Autodesk Inventor part; units mm, degrees
ref_plane "YZ Plane" through (0, 0, 0) normal (1, 0, 0) x (0, 1, 0)
ref_plane "XZ Plane" through (0, 0, 0) normal (0, 1, 0) x (-1, 0, 0)
ref_plane "XY Plane" through (0, 0, 0) normal (0, 0, 1) x (1, 0, 0)
sketch "Sketch1" plane through (0, 0, 0) normal (0, 1, 0) x (-1, 0, 0)
  point P0 (0, 0)
sketch "Sketch2" plane through (0, 0, 0) normal (0, 0, 1) x (1, 0, 0)
  line L0 (0, 0) -> (0, 25)
  line L1 (0, 25) -> (-5, 25)
  line L2 (-5, 25) -> (-5, 2.5)
  line L3 (-5, 2.5) -> (-85, 2.5)
  line L4 (-85, 2.5) -> (-85, 25)
  line L5 (-85, 25) -> (-90, 25)
  line L6 (-90, 25) -> (-90, 0)
  line L7 (-90, 0) -> (0, 0)
  line L8 (-85, 2.5) -> (-5, 2.5)
  line L9 (-5, 2.5) -> (-5, -2.5)
  line L10 (-5, -2.5) -> (-85, -2.5)
  line L11 (-85, -2.5) -> (-85, 2.5)
  dimension "d0" = 25
  dimension "d1" = 5
  dimension "d2" = 22.5
  dimension "d3" = 80
  dimension "d4" = 5
  dimension "d6" = 5
revolve "Revolution1" add sketch "Sketch2" angle 360 about axis through (-90, 0, 0) along (1, 0, 0) contours L7 L9 L2 L1 L0 | L7 L11 L3 L9 | L7 L6 L5 L4 L11
extrude "Extrusion1" add sketch "Sketch2" along normal mid plane 50 contours L9 L10 L11 L7 | L7 L11 L3 L9
sketch "Sketch3" plane through (-85, 2.5, -25) normal (0, 1, 0) x (1, 0, 0)
  line L0 (80, 0) -> (0, 0)
  line L1 (80, -49.8747) -> (80, -0.1253)
  line L2 (0, 0) -> (80, 0)
  line L3 (80, 0) -> (80, -49.8747)
  line L4 (80, -49.8747) -> (0, -49.8747)
  line L5 (0, -49.8747) -> (0, 0)
  line L6 (5, -5) -> (75, -5)
  line L7 (75, -5) -> (75, -44.8747)
  line L8 (75, -44.8747) -> (5, -44.8747)
  line L9 (5, -44.8747) -> (5, -5)
  point P0 (85, -25)
  dimension "d9" = 5
extrude "Extrusion2" cut sketch "Sketch3" against normal mid plane 20 contours L6 L7 L8 L9
properties part number "electronicsbay" material "ABS Plastic"
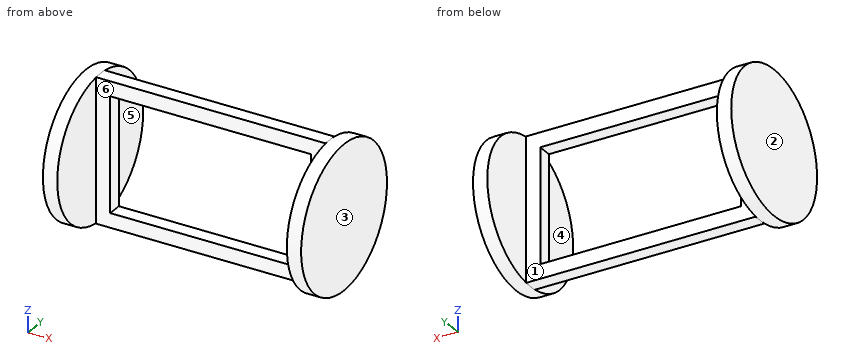
Input: part model. Units: mm. Frame: model coordinates. Face numbers are marked on the shaded views. A direction names the side the tool comes from. Give positions to 0.01 mm unless a question says otherwise; leave off trailing zeros. Write each loop counter-clockwise with the first axis right and the second up, starting at its lowest first coordinate (ties: lowest second). Pieces come first, ordered by that corner, then holes. Notation, with made-up numbers: M 12.5,65 L 37.5,65 A15 cw 37.5,72 Z; hole C 72.5,56 d6. An arc over 180 degrees is marked long. Use one line per item in the form item = value.
1. Reachability of the marked faces 5 and 6 from +Z, -Z, +X, -X, +Y, -Y: full face, straight path, thin tool, end or side. Return the list, or none.
Outcome:
face_5 = +Z, -Z, +Y
face_6 = +Z, -Z, -Y
2. Cut plane D-D on z = -15.5. Return loops of the section in (x, y), and give its area (3 significant figures).
Outcome:
outline = M -90,-19.62 L -85,-19.62 L -85,-2.5 L -80,-2.5 L -80,2.5 L -85,2.5 L -85,19.62 L -90,19.62 Z; M -10,-2.5 L -5,-2.5 L -5,-19.62 L 0,-19.62 L 0,19.62 L -5,19.62 L -5,2.5 L -10,2.5 Z
area = 442 mm²
3. First-contact query: P1, Ø3, axis at x = -47.5, z = 19.5, coming from the +Y side. Flat tip, straight axial feed; report the tip coordinate or a pass-through.
Outcome:
P1 = 2.5
4. Cut plane B-B on y = 7. Return loops of the section in (x, z), and give its area (3 significant figures).
Outcome:
outline = M -90,-24 L -85,-24 L -85,24 L -90,24 Z; M -5,-24 L 0,-24 L 0,24 L -5,24 Z
area = 480 mm²
5. Cut plane A-A on x = -47. Return loops of the section in (y, z), and give its area (3 significant figures).
Outcome:
outline = M -2.5,-25 L 2.5,-25 L 2.5,-20 L -2.5,-20 Z; M -2.5,19.87 L 2.5,19.87 L 2.5,25 L -2.5,25 Z
area = 50.6 mm²
6. Ray query, L1, parallel to X at y = -1, z = 10.5; L2, parallel to X at y = 18, z = 3; L3, parallel to Y at x = -84, z = 14. Return the intervals inside material, ascending.
Outcome:
L1 = -90 to -80, -10 to 0
L2 = -90 to -85, -5 to 0
L3 = -2.5 to 2.5
7. Cut plane C-C on z = 0. Return loops of the section in (x, y), and give its area (3 significant figures).
Outcome:
outline = M -90,-25 L -85,-25 L -85,-2.5 L -80,-2.5 L -80,2.5 L -85,2.5 L -85,25 L -90,25 Z; M -10,-2.5 L -5,-2.5 L -5,-25 L 0,-25 L 0,25 L -5,25 L -5,2.5 L -10,2.5 Z
area = 550 mm²
8. Mould query, pull axis X, two halves, no side actions, for the marked faces 1, 2, 3 and 4. Classes: released by +X, released by -X, zero draft, split by the parting line, or undercut.
Outcome:
face_1 = undercut
face_2 = released by -X
face_3 = released by +X
face_4 = undercut
